CAD build for the part. Positions are in the model's coordinates, mm. A direction names the side the tool comes from. Coordinates: 2 decimals unless noted, no trailing zeros. Order: outer loops, then holes, each group sorted by start corner. A loop starts at its lowest first (then second) coordinate and runs counter-clockwise, first axis right, second up. Notation, with made-up numbers: (-37, -18) - (-25, -18) arc R21 ccw to (-25, 18) - close; hole circle Ø11 at (47.5, 11). An arc over 180 degrees is marked (long way). Return JSON: item names as keys, results as strings.
from build123d import *

# Parameters (mm, degrees)
SKETCH2_R                    = 1.6500000000000001
CUT_EXTRUDE1_DEPTH           = 10
CHAMFER1_SIZE                = 0.5
CIRPATTERN1_COUNT            = 4
CHAMFER1_OF_CIRPATTERN1_SIZE = 0.5
CUT_EXTRUDE2_DEPTH           = 2
CHAMFER2_SIZE                = 1
SKETCH4_R                    = 1.09999999999999
CUT_EXTRUDE3_DEPTH           = 31.553232234904378
CHAMFER3_SIZE                = 1


# Read off the part's stored shape, not the designer's step: CirPattern2
with BuildPart() as part:
    # Sketch1 → Revolve1 (revolve)
    with BuildSketch(Plane(origin=(0, 0, 0), x_dir=(0, 0, -1), z_dir=(1, 0, 0))):
        Polygon((0, 0), (0, 21.5), (2, 21.5), (2, 20), (4.999999999999999, 20), (5.000000000000003, -1.7e-16), align=None)
    revolve(axis=Axis((0, -1.7e-16, -5.000000000000003), (0, 3e-17, 1)))

    # Sketch2 → Cut-Extrude1 (cut)
    with BuildSketch(Plane.XY):
        with Locations((0, 15)):
            Circle(SKETCH2_R)
    cut_extrude1 = extrude(amount=-CUT_EXTRUDE1_DEPTH, mode=Mode.SUBTRACT)

    # Chamfer1
    chamfer1_edges = [part.edges().sort_by_distance(p)[0] for p in [
        (-1.6500000000000001, 15.000000000000002, 0),
    ]]
    chamfer(chamfer1_edges, length=CHAMFER1_SIZE)

    # CirPattern1: Cut-Extrude1 ×4 about axis
    cirpattern1_axis = Axis((-2.619e-14, -5e-17, 0), (0, 0, 1))
    for i in range(1, CIRPATTERN1_COUNT):
        add(cut_extrude1.rotate(cirpattern1_axis, i * 360 / CIRPATTERN1_COUNT), mode=Mode.SUBTRACT)

    # Chamfer1 of CirPattern1
    chamfer1_of_cirpattern1_edges = [part.edges().sort_by_distance(p)[0] for p in [
        (-15.000000000000028, -1.649999999999973, 0),
        (1.649999999999946, -15.000000000000002, 0),
        (14.999999999999975, 1.6499999999999713, 0),
    ]]
    chamfer(chamfer1_of_cirpattern1_edges, length=CHAMFER1_OF_CIRPATTERN1_SIZE)

    # Sketch3 → Cut-Extrude2 (cut)
    with BuildSketch(Plane.XY):
        with BuildLine():
            ThreePointArc((-11.775069570500428, 11.77506957050046), (-11.77506957050042, 8.805221089516952), (-8.805221089516914, 8.805221089516971))
            Line((-8.805221089516925, 8.805221089516953), (-11.775069570500422, 11.77506957050046))
        make_face()
        with BuildLine():
            Line((-11.775069570500422, 11.77506957050046), (-8.805221089516925, 8.805221089516953))
            ThreePointArc((-8.805221089516914, 8.805221089516971), (-8.34999831173497, 9.486510122042029), (-8.190145330008676, 10.29014533000871))
            ThreePointArc((-8.190145330008676, 10.29014533000871), (-9.486510122041988, 12.230292348282413), (-11.775069570500428, 11.77506957050046))
        make_face()
    extrude(amount=-CUT_EXTRUDE2_DEPTH, mode=Mode.SUBTRACT)

    # Chamfer2
    chamfer2_edges = [part.edges().sort_by_distance(p)[0] for p in [
        (-11.775069570500419, 11.775069570500454, -2),
    ]]
    chamfer(chamfer2_edges, length=CHAMFER2_SIZE)

    # Sketch4 → Cut-Extrude3 (cut, through all)
    with BuildSketch(Plane.XY.offset(-2)):
        with Locations((-10.290145330008677, 10.29014533000871)):
            Circle(SKETCH4_R)
    extrude(amount=-CUT_EXTRUDE3_DEPTH, mode=Mode.SUBTRACT)

    # CirPattern2 outline → CirPattern2 (revolve, cut)
    with BuildSketch(Plane(origin=(10.29014533, -10.29014533, 0), x_dir=(1, 0, 0), z_dir=(0, -1, 0))):
        Polygon((1.1, -2), (2.1, -1), (2.1, 0), (0, 0), (0, -5), (1.1, -5), align=None)
    revolve(axis=Axis((10.29014533, -10.29014533, 0), (0, 0, 1)), mode=Mode.SUBTRACT)

    # Chamfer3
    chamfer3_edges = [part.edges().sort_by_distance(p)[0] for p in [
        (-2.45e-15, -20, -4.999999999999997),
    ]]
    chamfer(chamfer3_edges, length=CHAMFER3_SIZE)


solid = part.part
Item 1: Wall check: L1, parallel to Y at x = 0, z = -1.55; L2, parallel to X at y = 1.5, z = -3.35. Give the ranges that are in metal, low to high. Write a range as [from, to].
Findings below:
{"L1": "y = [-21.5, -16.65], [-13.35, 13.35], [16.65, 21.5]", "L2": "x = [-19.94, -15.69], [-14.31, 14.31], [15.69, 19.94]"}
Item 2: Mould opens along X. For faces 3 (the flat face through (0, 0, -5)), 4 (the cylindrical face through (10.017, -8.208, -0.493)), 5 (the cylindrical face through (-21.317, -2.799, -1.014)) say: released by +X, released by -X, zero draft, split by the parting line, or undercut.
Findings below:
{"face 3": "zero draft", "face 4": "undercut", "face 5": "split by the parting line"}
Item 3: Band-saw the part on C-C, the plane x = -1. Count the separate pieces of the cut face and the enclosed holes in it, then the cut area to 3 significant figures.
Findings below:
{"separate pieces": "3", "enclosed holes": "0", "area": "178 mm²"}
Item 4: Band-saw the part on B-B, the plane z = -3.1. List the corners of the cut face in (x, y), then the cut area to 3 significant figures.
Findings below:
{"outline": "circle Ø40 at (0, 0); hole circle Ø3.3 at (-15, 0); hole circle Ø2.2 at (-10.29, 10.29); hole circle Ø3.3 at (0, -15); hole circle Ø3.3 at (0, 15); hole circle Ø2.2 at (10.29, -10.29); hole circle Ø3.3 at (15, 0)", "area": "1,210 mm²"}
Item 5: Band-saw the part on A-A, the plane y = 0. List the corners of the cut face in (x, z), then the cut area to 4 significant figures.
Findings below:
{"outline": "(-21.5, -2) - (-20, -2) - (-20, -4) - (-19, -5) - (-16.65, -5) - (-16.65, -0.5) - (-17.15, 0) - (-21.5, 0) - close; (-13.35, -5) - (13.35, -5) - (13.35, -0.5) - (12.85, 0) - (-12.85, 0) - (-13.35, -0.5) - close; (16.65, -5) - (19, -5) - (20, -4) - (20, -2) - (21.5, -2) - (21.5, 0) - (17.15, 0) - (16.65, -0.5) - close", "area": "171.5 mm²"}
Item 6: Drop flat-ended pins along their axis: P1, Ø1, axis at y = 11.5, z = -4, coming from the +X side; P2, Ø1.5, axis at x = -15, z = -0.5, coming from the +Y side; P3, Ø3, axis at y = 8, z = -4.5, coming from the +X side. Give the stop position or say it passes through.
Findings below:
{"P1": "stops at x = 16.7", "P2": "stops at y = 16.1", "P3": "stops at x = 18.88"}
Item 7: Which spindle directions (+Z, -Z, +X, -X, +Y, -Y) get a long thin tool onto all of the face, cutting with end or side? Do faces 1 (the cylindrical face through (19.524, -4.336, -3.014)), 2 (the cylindrical face through (13.4, 0.4, -2.7)). Say none if no direction does.
Findings below:
{"face 1": "-Z", "face 2": "+Z, -Z"}
